Build history of the part. All positions in model axes, mm. Round coordinates to 2 decimals unless told otherwise and drop trailing zeros. Write each loop counter-clockwise with the first axis right and the second up, starting at its lowest first coordinate (ties: lowest second). Pieces come first, ordered by that corner, then holes. Notation, with made-up numbers: (19, -33.75) - (71, -33.75) arc R21 ccw to (71, 0.25) - close; hole circle Ø4 at (-36.75, -25.5). An arc over 180 degrees is marked (long way). Write each question's results on one line, items separated by ' | '.
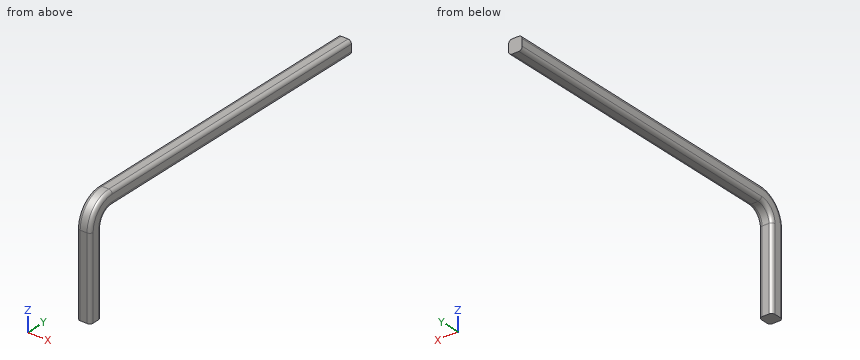
from build123d import *

# Parameters (mm, degrees)
F1_DEPTH = 12.7
F2_R     = 3.175


with BuildPart() as f1:
    # F0 (on Right) → F1 (new body)
    with BuildSketch(Plane.YZ):
        with BuildLine():
            Line((0, 76.2), (0, 0))
            Line((0, 0), (12.7, 0))
            Line((12.7, 0), (12.7, 76.2))
            ThreePointArc((12.7, 76.2), (16.419744, 85.180256), (25.4, 88.9))
            Line((25.4, 88.9), (304.8, 88.9))
            Line((304.8, 88.9), (304.8, 101.6))
            Line((304.8, 101.6), (25.4, 101.6))
            ThreePointArc((25.4, 101.6), (7.439488, 94.160512), (0, 76.2))
        make_face()
    extrude(amount=F1_DEPTH)

    # F2
    f2_edges = [f1.edges().sort_by_distance(p)[0] for p in [
        (12.7, 7.439488, 94.160512),
        (12.7, 165.1, 88.9),
        (0, 165.1, 101.6),
        (0, 165.1, 88.9),
    ]]
    fillet(f2_edges, radius=F2_R)


solid = f1.part
(1) Slice it at B-B, the plane y = 207.5. Write the cut outline in (x, z) (3 decimals), and give its area (3 significant figures).
Worked answers:
outline: (0, 92.075) arc R3.175 ccw to (3.175, 88.9) - (9.525, 88.9) arc R3.175 ccw to (12.7, 92.075) - (12.7, 98.425) arc R3.175 ccw to (9.525, 101.6) - (3.175, 101.6) arc R3.175 ccw to (0, 98.425) - close | area: 153 mm2
(2) Drill centre lines: probe 1 along Y at (x, z) = (8.75, 58.5); probe 2 along Z at (x, y) = (3.25, 193); probe 3 along Y at (x, z) = (5, 96). Where is each one in solid material? Low to high. Write a range as [from, to].
Worked answers:
probe 1: y = [0, 12.7] | probe 2: z = [88.9, 101.6] | probe 3: y = [9.49, 304.8]
(3) Flat gauge pins, fed straight in: pin 1 Ø3 at (x, z) = (9.5, 32) entering from +Y; pin 2 Ø1.9 at (x, y) = (7.5, 180.5) entering from -Z; pin 3 Ø5 at (x, z) = (7.5, 81) entering from +Y. Where does each tip first touch, or does it go through?
Worked answers:
pin 1: stops at y = 12.7 | pin 2: stops at z = 88.9 | pin 3: stops at y = 15.01
(4) Slice it at A-A, the plane z = 69. Write the cut outline in (x, y) (3 decimals).
Worked answers:
outline: (0, 3.175) arc R3.175 ccw to (3.175, 0) - (9.525, 0) arc R3.175 ccw to (12.7, 3.175) - (12.7, 9.525) arc R3.175 ccw to (9.525, 12.7) - (3.175, 12.7) arc R3.175 ccw to (0, 9.525) - close
